from build123d import *

# Parameters (mm, degrees)
PAD038_DEPTH    = 3
SKETCH068_W     = 4
SKETCH068_H     = 13.628868
PAD039_DEPTH    = 10
SKETCH070_W     = 16.3
SKETCH070_H     = 2.6
POCKET031_DEPTH = 11
SKETCH071_W     = 16
SKETCH071_H     = 2.72
POCKET032_DEPTH = 4
SKETCH078_W     = 22.244752
SKETCH078_H     = 7.861252
POCKET037_DEPTH = 2
SKETCH081_W     = 13.416131
SKETCH081_H     = 2.3
PAD042_DEPTH    = 1.5
SKETCH082_W     = 13.368385
SKETCH082_H     = 2.3
PAD043_DEPTH    = 1.5
SKETCH083_W     = 2.761169
SKETCH083_H     = 2.284319
PAD044_DEPTH    = 0.5
SKETCH084_W     = 2.757059
SKETCH084_H     = 2.258492
PAD045_DEPTH    = 0.5
CHAMFER014_SIZE = 1.4
FILLET012_R     = 3
SKETCH086_R     = 1.2
POCKET038_DEPTH = 2
SKETCH087_R     = 0.7
POCKET039_DEPTH = 5
CHAMFER017_SIZE = 1


with BuildPart() as part:
    # Sketch069 → Pad038 (new body)
    with BuildSketch(Plane.XY.offset(-8.2)):
        Polygon((24.588766, -45.296032), (-24.588766, -45.296032), (-30.301265, -31.40278), (-26.329521, -31.40278), (-26.329521, -26.47687), (-30.301265, -26.47687), (-30.301265, -16.823771), (-37.665775, -16.823771), (-37.665775, -30.675779), (-35.365035, -37.426579), (-33.111649, -43.283928), (-30.227776, -48.090385), (-25.709705, -52.800713), (-24.427355, -56.731705), (25.394418, -56.731705), (25.709705, -52.800713), (30.227776, -48.090385), (33.111649, -43.283928), (35.365035, -37.426579), (37.665775, -30.675779), (37.665775, -16.823771), (30.301265, -16.823771), (30.301265, -26.47687), (26.329521, -26.47687), (26.329521, -31.40278), (30.301265, -31.40278), align=None)
    extrude(amount=-PAD038_DEPTH)

    # Sketch068 → Pad039 (join)
    with BuildSketch(Plane.XY.offset(-8.2)):
        Polygon((33.602105, -16.851452), (33.602105, -30.48032), (32.974419, -36.715145), (31.524649, -42.567276), (29.661472, -46.157772), (27.526943, -48.830738), (24.790402, -50.266937), (0, -50.266937), (0, -56.462727), (25.154314, -56.462727), (25.588615, -52.727741), (30.133654, -48.083988), (32.913181, -43.219818), (35.345268, -36.850067), (37.602105, -30.48032), (37.602105, -16.851452), align=None)
        with Locations((-35.602105, -23.665886)):
            Rectangle(SKETCH068_W, SKETCH068_H)
    extrude(amount=PAD039_DEPTH)

    # Sketch070 (on Face5 of Pad039) → Pocket031 (cut)
    with BuildSketch(Plane(origin=(0, 0, -11.2), x_dir=(1, 0, 0), z_dir=(0, 0, -1))):
        with Locations((9.95, 53.3)):
            Rectangle(SKETCH070_W, SKETCH070_H)
    extrude(amount=-POCKET031_DEPTH, mode=Mode.SUBTRACT)

    # Sketch071 (on Face35 of Pocket031) → Pocket032 (cut)
    with BuildSketch(Plane(origin=(0, -50.266937, 0), x_dir=(-1, 0, 0), z_dir=(0, 1, 0))):
        with Locations((-9.86, -0.26)):
            Rectangle(SKETCH071_W, SKETCH071_H)
    extrude(amount=-POCKET032_DEPTH, mode=Mode.SUBTRACT)

    # Sketch078 (on Face53 of Pocket032) → Pocket037 (cut)
    with BuildSketch(Plane.XY.offset(1.8)):
        with Locations((10.750455, -53.658291)):
            Rectangle(SKETCH078_W, SKETCH078_H)
    extrude(amount=-POCKET037_DEPTH, mode=Mode.SUBTRACT)

    # Sketch081 (on Face45 of Pocket037) → Pad042 (join)
    with BuildSketch(Plane.YZ.offset(-33.602105)):
        with Locations((-23.705268, -1.15)):
            Rectangle(SKETCH081_W, SKETCH081_H)
    extrude(amount=PAD042_DEPTH)

    # Sketch082 (on Face29 of Pad042) → Pad043 (join)
    with BuildSketch(Plane(origin=(33.602105, 0, 0), x_dir=(0, -1, 0), z_dir=(-1, 0, 0))):
        with Locations((23.672373, -1.15)):
            Rectangle(SKETCH082_W, SKETCH082_H)
    extrude(amount=PAD043_DEPTH)

    # Sketch083 (on Face68 of Pad043) → Pad044 (join)
    with BuildSketch(Plane(origin=(32.102105, 0, 0), x_dir=(0, -1, 0), z_dir=(-1, 0, 0))):
        with Locations((18.510706, -1.142159)):
            Rectangle(SKETCH083_W, SKETCH083_H)
    extrude(amount=PAD044_DEPTH)

    # Sketch084 (on Face70 of Pad044) → Pad045 (join)
    with BuildSketch(Plane.YZ.offset(-32.102105)):
        with Locations((-18.51388, -1.146782)):
            Rectangle(SKETCH084_W, SKETCH084_H)
    extrude(amount=PAD045_DEPTH)

    # Chamfer014
    chamfer014_edges = [part.edges().sort_by_distance(p)[0] for p in [
        (33.602105, -23.672373, -2.3),
        (-33.602105, -23.705268, -2.3),
    ]]
    chamfer(chamfer014_edges, length=CHAMFER014_SIZE)

    # Fillet012
    fillet012_edges = [part.edges().sort_by_distance(p)[0] for p in [
        (37.602105, -23.665886, 1.8),
        (-37.602105, -23.665886, 1.8),
    ]]
    fillet(fillet012_edges, radius=FILLET012_R)

    # Sketch086 (on Face4 of Fillet012) → Pocket038 (cut)
    with BuildSketch(Plane.XY.offset(-8.2)):
        with Locations((-28.5, -29.067181)):
            Circle(SKETCH086_R)
        with Locations((28.5, -29.067181)):
            Circle(SKETCH086_R)
        with Locations((-21, -47.610665)):
            Circle(SKETCH086_R)
        with Locations((21, -47.610665)):
            Circle(SKETCH086_R)
    extrude(amount=-POCKET038_DEPTH, mode=Mode.SUBTRACT)

    # Sketch087 (on Face63 of Pocket038) → Pocket039 (cut)
    with BuildSketch(Plane.XY.offset(-10.2)):
        with Locations((-28.5, -29.054167)):
            Circle(SKETCH087_R)
        with Locations((28.5, -29.054167)):
            Circle(SKETCH087_R)
        with Locations((-21, -47.60955)):
            Circle(SKETCH087_R)
        with Locations((21, -47.60955)):
            Circle(SKETCH087_R)
    extrude(amount=-POCKET039_DEPTH, mode=Mode.SUBTRACT)

    # Chamfer017
    chamfer017_edges = [part.edges().sort_by_distance(p)[0] for p in [
        (30.301265, -21.65032, -8.2),
        (27.445016, -38.349406, -8.2),
        (0, -45.296032, -8.2),
        (-27.445016, -38.349406, -8.2),
        (-30.301265, -21.65032, -8.2),
    ]]
    chamfer(chamfer017_edges, length=CHAMFER017_SIZE)


solid = part.part
Input: part model. Units: mm. Frame: model coordinates. A direction names the side the tool comes from. Give positions to 0.01 mm unless a question says otherwise; leave off trailing zeros. Order: outer loops, then holes, each group sorted by start corner. A loop starts at its lowest first (then second) coordinate and runs counter-clockwise, first axis right, second up. Notation, with made-up numbers: (73.5, 12.25) -> (101.5, 12.25) arc R31 ccw to (101.5, 39.25) -> close; hole circle Ø10 at (41.25, 18.25). An arc over 180 degrees is marked (long way). Use one line per item in the form item = value.
1) Mould query, pull axis Y, two halves, no side actions, for faces 4 (the flat face through (17.86, -51, -1)), 5 (the flat face through (-33, -16.997, -1)), 6 (the flat face through (-27.405, -38.447, -10.186)), 7 (the flat face through (34.22, -40.4, -9.68)). Classes: pulls with the +Y half, pulls with the -Y half, needs draft (parallel to the pull), parting line crosses it, or undercut.
Response values:
face_4 = needs draft
face_5 = pulls with the +Y half
face_6 = undercut
face_7 = pulls with the -Y half
2) Line query: probe 1 along Y at (x, z) = (-21, -9.4); probe 2 along X at (y, z) = (-26.5, -6.75); probe 3 along X at (y, z) = (-47, -9.5). Output: solid intervals per line, ascending.
Response values:
probe_1 = -56.73 to -48.81, -46.41 to -45.3
probe_2 = -37.6 to -33.6, 33.6 to 37.6
probe_3 = -30.88 to -22.03, -19.97 to 19.97, 22.03 to 30.88
3) Section C-C, the plane x = 21. Return loops of the section in (y, z), and give its area (3 significant figures).
Response values:
outline = (-56.73, -11.2) -> (-48.31, -11.2) -> (-48.31, -10.2) -> (-48.81, -10.2) -> (-48.81, -8.2) -> (-50.27, -8.2) -> (-50.27, -0.2) -> (-56.46, -0.2) -> (-56.46, -8.2) -> (-56.73, -8.2) -> close; (-46.91, -11.2) -> (-45.3, -11.2) -> (-45.3, -9.2) -> (-46.3, -8.2) -> (-46.41, -8.2) -> (-46.41, -10.2) -> (-46.91, -10.2) -> close
area = 77.2 mm^2
4) Reachability of faces 1 (the flat face through (0, -53, -4)), 2 (the flat face through (1.86, -51, -1)), 3 (the flat face through (-33, -30.413, -1)) from +Z, -Z, +X, -X, +Y, -Y: full face, straight path, thin tool, end or side. Return the list, or none.
Response values:
face_1 = +Z, -X, +Y, -Y
face_2 = +Z, +Y
face_3 = +Z, -Y
5) First-contact query: pin 1 Ø1.2 at (y, z) = (-23.5, -1.5) entering from -X; pin 2 Ø1 at (x, z) = (4, -2.5) entering from +Y; pin 3 Ø4 at (x, z) = (5, -8.5) entering from +Y. Flat tips, straight axial feed; report the tip coordinate or a pass-through.
Response values:
pin_1 = -37.6
pin_2 = -50.27
pin_3 = -45.3
6) Section D-D, the plane x = -28.5. Return loops of the section in (y, z).
Response values:
outline = (-49.89, -11.2) -> (-35.78, -11.2) -> (-35.78, -9.2) -> (-38.41, -8.2) -> (-49.89, -8.2) -> close; (-31.4, -11.2) -> (-29.75, -11.2) -> (-29.75, -10.2) -> (-30.27, -10.2) -> (-30.27, -8.2) -> (-31.4, -8.2) -> close; (-28.35, -11.2) -> (-26.48, -11.2) -> (-26.48, -8.2) -> (-27.87, -8.2) -> (-27.87, -10.2) -> (-28.35, -10.2) -> close
7) Section A-A, the plane z = -5. Return loops of the section in (x, y), and give its area (3 significant figures).
Response values:
outline = (-37.6, -30.48) -> (-33.6, -30.48) -> (-33.6, -16.85) -> (-37.6, -16.85) -> close; (0, -56.46) -> (25.15, -56.46) -> (25.59, -52.73) -> (30.13, -48.08) -> (32.91, -43.22) -> (35.35, -36.85) -> (37.6, -30.48) -> (37.6, -16.85) -> (33.6, -16.85) -> (33.6, -30.48) -> (32.97, -36.72) -> (31.52, -42.57) -> (29.66, -46.16) -> (27.53, -48.83) -> (24.79, -50.27) -> (0, -50.27) -> close; hole (1.8, -54.6) -> (18.1, -54.6) -> (18.1, -52) -> (1.8, -52) -> close
area = 274 mm^2
